from build123d import *

# Parameters (mm, degrees)
SCHIZZO1_W                   = 4.5
SCHIZZO1_H                   = 3.825
SCHIZZO1_H_2                 = 4.475
SCHIZZO1_W_2                 = 4.1
ESTRUSIONE_ESTRUSIONE1_DEPTH = 6.6
SCHIZZO1_4_W                 = 4.5
SCHIZZO1_4_H                 = 4.475
SCHIZZO1_4_H_2               = 3.825
SCHIZZO1_4_W_2               = 10.65
SCHIZZO1_4_W_3               = 4.1
ESTRUSIONE_ESTRUSIONE2_DEPTH = 0.4


with BuildPart() as part:
    # Schizzo1 → Estrusione-Estrusione1 (new body)
    with BuildSketch(Plane.XZ.offset(-9.997150898)):
        with Locations((-38.335959006, 140.797368204)):
            Rectangle(SCHIZZO1_W, SCHIZZO1_H)
        with Locations((-38.335959006, 136.647368204)):
            Rectangle(SCHIZZO1_W, SCHIZZO1_H_2)
        with Locations((-23.385959006, 140.797368204)):
            Rectangle(SCHIZZO1_W_2, SCHIZZO1_H)
    extrude(amount=-ESTRUSIONE_ESTRUSIONE1_DEPTH)

    # Schizzo1<4> → Estrusione-Estrusione2 (add)
    with BuildSketch(Plane.XZ.offset(-9.997150898)):
        with Locations((-38.335959006, 136.647368204)):
            Rectangle(SCHIZZO1_4_W, SCHIZZO1_4_H)
        with Locations((-38.335959006, 140.797368204)):
            Rectangle(SCHIZZO1_4_W, SCHIZZO1_4_H_2)
        with Locations((-30.760959006, 140.797368204)):
            Rectangle(SCHIZZO1_4_W_2, SCHIZZO1_4_H_2)
        with Locations((-23.385959006, 140.797368204)):
            Rectangle(SCHIZZO1_4_W_3, SCHIZZO1_4_H_2)
    extrude(amount=-ESTRUSIONE_ESTRUSIONE2_DEPTH)


solid = part.part
Geometry: final body of the model. Coordinates: model frame, mm. A direction names the side the tool comes from. Round coordinates to 2 decimals unless told otherwise and drop trailing zeros. Loops run counter-clockwise (first coordinate to the right, second up) from the corner with the lowest first, then second, coordinate; pieces in that order, holes last. Notation, with made-up numbers: (19, 89.5) -> (59, 89.5) arc R23 ccw to (59, 101.5) -> close; hole circle Ø4 at (69, -11.5). An arc over 180 degrees is marked (long way). One line per question, with ' | ' between items. Start each with the question number.
1. Contact query for a flat-ended pin moving along its axis: pin 1 (1.1 mm diameter, centred on x = -31, z = 140, fed in from +Y). Output: stop coordinate, or through.
2. Section D-D on z = 138.5. Output: boundary loops of the cut face in (x, y).
3. Section C-C on x = -34. Output: boundary loops of the cut face in (y, z), and give its area (3 significant figures).
4. Section A-A on y = 12. Output: boundary loops of the cut face in (x, z).
5. Set-up query: faces 1 (the face through (-25.436, 13, 141)), 2 (the face through (-21.336, 13, 141)). Return all of +Z, -Z, +X, -X, +Y, -Y with unobstructed straight access to the full face (end or side cutting, diameter ignored); none if empty.
6. Mould query, pull axis X, two halves, no side actions, for faces 3 (the face through (-36.086, 13, 139)), 4 (the face through (-40.586, 13, 139)), 5 (the face through (-25, 13, 138.885)). Classes: pulls with the +X half, pulls with the -X half, needs draft (parallel to the pull), parting line crosses it, or undercut.
7. Line query: line 1 along X through (y, z) = (12, 142.25); line 2 along X through (y, z) = (13.5, 137); line 3 along Y through (x, z) = (-32.25, 140.5). Output: solid intervals per line, ascending. Write a range as [from, to].
8. Section B-B on z = 140.5. Output: boundary loops of the cut face in (x, y), and give its area (3 significant figures).
Returned:
1) pin 1: stops at y = 10.4
2) outline: (-40.59, 10) -> (-36.09, 10) -> (-36.09, 16.6) -> (-40.59, 16.6) -> close
3) outline: (10, 138.88) -> (10.4, 138.88) -> (10.4, 142.71) -> (10, 142.71) -> close | area: 1.53 mm2
4) outline: (-40.59, 134.41) -> (-36.09, 134.41) -> (-36.09, 142.71) -> (-40.59, 142.71) -> close; (-25.44, 138.88) -> (-21.34, 138.88) -> (-21.34, 142.71) -> (-25.44, 142.71) -> close
5) face 1: +Z, -Z, +Y | face 2: +Z, -Z, +X, +Y, -Y
6) face 3: undercut | face 4: pulls with the -X half | face 5: needs draft
7) line 1: x = [-40.59, -36.09], [-25.44, -21.34] | line 2: x = [-40.59, -36.09] | line 3: y = [10, 10.4]
8) outline: (-40.59, 10) -> (-21.34, 10) -> (-21.34, 16.6) -> (-25.44, 16.6) -> (-25.44, 10.4) -> (-36.09, 10.4) -> (-36.09, 16.6) -> (-40.59, 16.6) -> close | area: 61.0 mm2
